Read the model definition and answer for the solid it produces. Units are mm, in the model's axes. Coordinates: 2 decimals unless noted, no trailing zeros. Order: outer loops, then holes, each group sorted by start corner. A loop starts at its lowest first (then second) coordinate and runs counter-clockwise, first axis right, second up. Notation, with made-up numbers: (74.5, -31) -> (80.5, -31) arc R19 cw to (80.5, 0) -> close; hole circle Ø2 at (1.25, 77.25). An arc over 180 degrees is marked (long way). Answer in a Markdown table with one row per item.
from build123d import *

# Parameters (mm, degrees)
SKETCH1_W           = 82.55
SKETCH1_H           = 82.55
BOSS_EXTRUDE1_DEPTH = 3.175
SKETCH2_W           = 25.4
SKETCH2_H           = 25.4
SKETCH2_W_2         = 19.05
SKETCH2_H_2         = 3.175
SKETCH2_W_3         = 3.175
SKETCH2_H_3         = 19.05
CUT_EXTRUDE1_DEPTH  = 3.175
SKETCH3_W           = 19.05
SKETCH3_H           = 3.175
SKETCH3_W_2         = 3.175
SKETCH3_H_2         = 19.05
CUT_EXTRUDE2_DEPTH  = 3.175


with BuildPart() as part:
    # Sketch1 → Boss-Extrude1 (new body)
    with BuildSketch(Plane(origin=(0, 0, 0), x_dir=(1, 0, 0), z_dir=(0, 1, 0))):
        with Locations((41.275, 41.275)):
            Rectangle(SKETCH1_W, SKETCH1_H)
    extrude(amount=BOSS_EXTRUDE1_DEPTH)

    # Sketch2 → Cut-Extrude1 (cut)
    with BuildSketch(Plane(origin=(0, 3.175, 0), x_dir=(1, 0, 0), z_dir=(0, 1, 0))):
        with Locations((41.275, 41.275)):
            Rectangle(SKETCH2_W, SKETCH2_H)
        with Locations((41.275, 68.2625)):
            Rectangle(SKETCH2_W_2, SKETCH2_H_2)
        with Locations((14.2875, 41.275)):
            Rectangle(SKETCH2_W_3, SKETCH2_H_3)
        with Locations((68.2625, 41.275)):
            Rectangle(SKETCH2_W_3, SKETCH2_H_3)
        with Locations((41.275, 14.2875)):
            Rectangle(SKETCH2_W_2, SKETCH2_H_2)
    extrude(amount=-CUT_EXTRUDE1_DEPTH, mode=Mode.SUBTRACT)

    # Sketch3 → Cut-Extrude2 (cut)
    with BuildSketch(Plane(origin=(0, 3.175, 0), x_dir=(1, 0, 0), z_dir=(0, 1, 0))):
        with Locations((41.275, 80.9625)):
            Rectangle(SKETCH3_W, SKETCH3_H)
        with Locations((80.9625, 41.275)):
            Rectangle(SKETCH3_W_2, SKETCH3_H_2)
        with Locations((41.275, 1.5875)):
            Rectangle(SKETCH3_W, SKETCH3_H)
        with Locations((1.5875, 41.275)):
            Rectangle(SKETCH3_W_2, SKETCH3_H_2)
    extrude(amount=-CUT_EXTRUDE2_DEPTH, mode=Mode.SUBTRACT)


solid = part.part
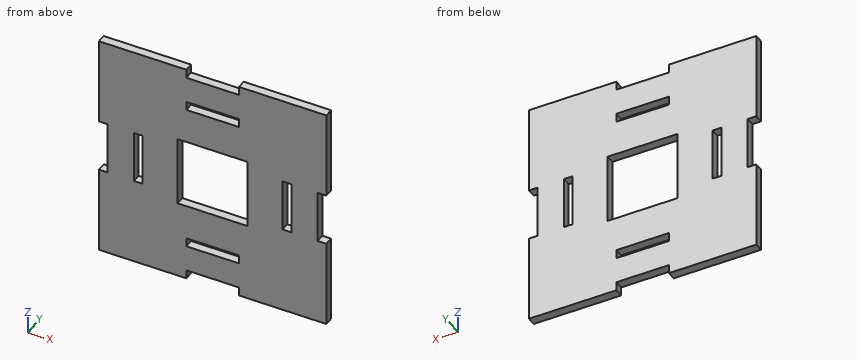
Q1. The part is cut by section C-C (z = -33.5). Write down the section's boundary in (x, y) (3 decimals), then the cut area to 3 significant figures.
Outcome:
| item | result |
|---|---|
| outline | (3.175, 0) -> (12.7, 0) -> (12.7, 3.175) -> (3.175, 3.175) -> close; (15.875, 0) -> (28.575, 0) -> (28.575, 3.175) -> (15.875, 3.175) -> close; (53.975, 0) -> (66.675, 0) -> (66.675, 3.175) -> (53.975, 3.175) -> close; (69.85, 0) -> (79.375, 0) -> (79.375, 3.175) -> (69.85, 3.175) -> close |
| area | 141 mm² |
Q2. Given pin 1 (1.6 mm diameter, centred on y = 1.5, z = -39, fed in from -X) (3 decimals); pin 2 (1.6 mm diameter, centred on y = 1.5, z = -81.5, fed in from -X); pin 3 (1 mm diameter, centred on x = 35, y = 1, fed in from -Z) (3 decimals); pin 4 (1 mm diameter, centred on y = 1, z = -43.5, fed in from +X) (3 decimals), each flat-ended and moving along its own axis, determine where each tip first touches the part or whether it passes through.
Outcome:
| item | result |
|---|---|
| pin 1 | x = 3.175 |
| pin 2 | x = 0 |
| pin 3 | z = -79.375 |
| pin 4 | x = 79.375 |
Q3. The part is cut by section B-B (x = 44). Write down the section's boundary in (y, z) (3 decimals).
Outcome:
| item | result |
|---|---|
| outline | (0, -79.375) -> (3.175, -79.375) -> (3.175, -69.85) -> (0, -69.85) -> close; (0, -66.675) -> (3.175, -66.675) -> (3.175, -53.975) -> (0, -53.975) -> close; (0, -28.575) -> (3.175, -28.575) -> (3.175, -15.875) -> (0, -15.875) -> close; (0, -12.7) -> (3.175, -12.7) -> (3.175, -3.175) -> (0, -3.175) -> close |
Q4. The part is cut by section D-D (y = 2.6). Give the number of separate pieces and of enclosed holes in the cut face, then the cut area to 3 significant figures.
Outcome:
| item | result |
|---|---|
| separate pieces | 1 |
| enclosed holes | 5 |
| area | 5,690 mm² |
Q5. Consider line 1 (Z direction, x = 40.5, y = 0.5) (3 decimals); line 2 (X direction, y = 0.3, z = -42.5) (3 decimals); line 3 (Z direction, x = 31, y = 1.85) (3 decimals). Determine where each line is inside the solid, lowest interval first.
Outcome:
| item | result |
|---|---|
| line 1 | -79.375 to -69.85, -66.675 to -53.975, -28.575 to -15.875, -12.7 to -3.175 |
| line 2 | 3.175 to 12.7, 15.875 to 28.575, 53.975 to 66.675, 69.85 to 79.375 |
| line 3 | -82.55 to -53.975, -28.575 to 0 |
Q6. The part is cut by section A-A (z = -53). Write down the section's boundary in (x, y) (3 decimals).
Outcome:
| item | result |
|---|---|
| outline | (0, 0) -> (28.575, 0) -> (28.575, 3.175) -> (0, 3.175) -> close; (53.975, 0) -> (82.55, 0) -> (82.55, 3.175) -> (53.975, 3.175) -> close |
